CAD build for the part. Positions are in the model's coordinates, mm. A direction names the side the tool comes from. Round coordinates to 2 decimals unless told otherwise and drop trailing zeros. Write each loop counter-clockwise with the first axis right and the second up, starting at its lowest first coordinate (ties: lowest second). Pieces come first, ordered by that corner, then holes. Notation, with made-up numbers: (53, 43) - (83, 43) arc R24 cw to (83, 71) - close; hole circle Ø6 at (73.25, 75.5). An arc over 180 degrees is marked (long way). Put each result on its own line as item: value. Start each with the question number.
Item 1: Cut at A-A (z = 9). Give the cut face in (x, y).
Item 2: Pin check, flat tips, straight feed: pin 1 Ø1 at (y, z) = (0.5, 3) entering from +X; pin 2 Ø2 at (x, z) = (-24.5, -11.5) entering from -Y; pin 3 Ø4.5 at (x, y) = (2, -2.5) entering from -Z. Stop position of each tip, or through.
Item 3: 3-axis set-ups, long thin cutter, end or side, ignore diameter. For faces 1 (the flat face through (-10.573, -2, 9)), 2 (the flat face through (70, 10, 0)), 3 (the flat face through (10.573, -2, 9)), 4 (the flat face through (0, -2, 12.433)), 5 (the flat face through (0, -2, 5)): which of +Z, -Z, +X, -X, +Y, -Y reach the whole face in a straight line?
Item 4: Cut at D-D (x = -52.5). Give the cut face in (y, z), and give its area (3 significant figures).
Item 5: Cut at B-B (x = -5). Give the cut face in (y, z).
Item 6: Drill centre lines: line 1 (Y direction, x = -46, z = 6); line 2 (X direction, y = -0.5, z = 11); line 3 (X direction, y = 16, z = -19). Where is each one in solid material? Low to high. Write a range as from..to.
Item 7: Cut at C-C (z = -0.5). Give the cut face in (x, y), and give its area (3 significant figures).
```python
from build123d import *

# Parameters (mm, degrees)
SKETCH_1_W      = 140
SKETCH_1_H      = 42
EXTRUDE_1_DEPTH = 20
SKETCH_2_W      = 21.145082228
SKETCH_2_H      = 7.433476263
EXTRUDE_2_DEPTH = 4
FILLET_1_R      = 5
FILLET_2_R      = 5


with BuildPart() as part:
    # 草图1 → 凸台-拉伸1 (new body)
    with BuildSketch(Plane(origin=(0, 0, 0), x_dir=(1, 0, 0), z_dir=(0, 1, 0))):
        Rectangle(SKETCH_1_W, SKETCH_1_H)
    extrude(amount=EXTRUDE_1_DEPTH)

    # 草图2 → 凸台-拉伸2 (add)
    with BuildSketch(Plane.XZ):
        with Locations((0, 8.716738132)):
            Rectangle(SKETCH_2_W, SKETCH_2_H)
    extrude(amount=EXTRUDE_2_DEPTH)

    # 圆角1
    fillet_1_edges = [part.edges().sort_by_distance(p)[0] for p in [
        (-70, 20, 0),
        (70, 20, 0),
    ]]
    fillet(fillet_1_edges, radius=FILLET_1_R)

    # 圆角2
    fillet_2_edges = [part.edges().sort_by_distance(p)[0] for p in [
        (-70, 0, 0),
        (70, 0, 0),
    ]]
    fillet(fillet_2_edges, radius=FILLET_2_R)


solid = part.part
```
Output values:
1. outline: (-70, 5) arc R5 ccw to (-65, 0) - (-10.57, 0) - (-10.57, -4) - (10.57, -4) - (10.57, 0) - (65, 0) arc R5 ccw to (70, 5) - (70, 15) arc R5 ccw to (65, 20) - (-65, 20) arc R5 ccw to (-70, 15) - close
2. pin 1: x = 68
2. pin 2: y = 0
2. pin 3: z = 5
3. face 1: +Z, -Z, -X, -Y
3. face 2: +Z, -Z, +X, +Y, -Y
3. face 3: +Z, -Z, +X, -Y
3. face 4: +Z, +X, -X, -Y
3. face 5: -Z, +X, -X, -Y
4. outline: (0, -21) - (20, -21) - (20, 21) - (0, 21) - close
4. area: 840 mm2
5. outline: (-4, 5) - (0, 5) - (0, -21) - (20, -21) - (20, 21) - (0, 21) - (0, 12.43) - (-4, 12.43) - close
6. line 1: 0..20
6. line 2: -10.57..10.57
6. line 3: -69.9..69.9
7. outline: (-70, 5) arc R5 ccw to (-65, 0) - (65, 0) arc R5 ccw to (70, 5) - (70, 15) arc R5 ccw to (65, 20) - (-65, 20) arc R5 ccw to (-70, 15) - close
7. area: 2,780 mm2
